Input: part model. Units: mm. Frame: model coordinates. A direction names the side the tool comes from. Coordinates: 2 decimals unless noted, no trailing zeros. Loops run counter-clockwise (first coordinate to the right, second up) from the corner with the lowest first, then second, coordinate; pieces in that order, holes last. Notation, with made-up numbers: (49, 57) - (92, 57) arc R22 cw to (92, 72) - close; hole circle Ø1 at (5.25, 78.5). An arc over 180 degrees is marked (long way). Use a Markdown table: item, result. Add a question column.
1. Ray query, L1, parallel to Z at x = 63, y = -8.25; L2, parallel to Y at x = 30.5, z = -8.5; L3, parallel to Z at x = -11.5, y = -5. Return the intervals inside material, ascending. Write a range as [from, to].
2. Section query C-C on z = 6. Return the cut outline in (x, y).
3. Contact query for flat-ended pins moving along their axis: P1, Ø3, axis at x = -13.5, y = -9.5, coming from the +Z side; P2, Ø1.5, axis at x = -59.09, z = -20.84, coming from the +Y side; P3, Ø7, axis at x = -11, y = -9, coming from the -Z side; P4, Ø17, axis at x = 19.5, z = -5, coming from the -Y side. Output: stop coordinate, or through.
4. Access query for faces 1 (the face through (10, -9, 16.801)), 2 (the face through (10, -6.35, 40)), 3 (the face through (10, 2, -22.216)). Directions: +Z, -Z, +X, -X, +Y, -Y. A direction counts if a zero-diameter tool reaches every point of the face in a straight line with its end or side. Return the directions, or none.
5. Section query B-B on y = -10.5. Return the cut outline in (x, z), then the cut area to 3 significant figures.
6. Section query A-A on x = 20.5. Return the cut outline in (y, z).
```python
from build123d import *

# Parameters (mm, degrees)
F0_W        = 142.24
F0_H        = 80.9625
F0_R        = 0.635
F1_DEPTH    = 6.35
F2_T1_DEPTH = 168.3682991577
F3_W        = 142.24
F3_H        = 9.525
F4_DEPTH    = 6.35


# Not quite as in the source:
# - a fillet or chamfer that OpenCascade refuses, or shapes differently, is made with other operations: its cross-section is extruded or revolved along the edge and cut away or added


with BuildPart() as f1:
    # F0 (on Front) → F1 (new body, symmetric)
    with BuildSketch(Plane.XZ):
        with Locations((10.6546021998, 18.2648575297)):
            Rectangle(F0_W, F0_H)
        with Locations((-59.0889267623, -20.8356846124)):
            Circle(F0_R, mode=Mode.SUBTRACT)
        with Locations((80.2197679877, -20.9288131446)):
            Circle(F0_R, mode=Mode.SUBTRACT)
        with Locations((-58.7598197162, 57.2748109698)):
            Circle(F0_R, mode=Mode.SUBTRACT)
        with Locations((80.3315266967, 57.7001310885)):
            Circle(F0_R, mode=Mode.SUBTRACT)
    extrude(amount=F1_DEPTH, both=True)

    # F2: chamfer of 5.08 on 2 edges, made by hand

    # F2_s2 → F2_t1 (cut)
    with BuildSketch(Plane.YZ.offset(-73.5295473791)):
        Polygon((-1.27, -22.2163924703), (-6.35, -17.1363924703), (-6.35, -22.2163924703), align=None)
        Polygon((-1.27, 58.7461075297), (-6.35, 53.6661075297), (-6.35, 58.7461075297), align=None)
    extrude(amount=F2_T1_DEPTH, mode=Mode.SUBTRACT)

    # F3 (on face) → F4 (join)
    with BuildSketch(Plane.XZ.offset(6.35)):
        with Locations((10.6546021998, 21.5639811352)):
            Rectangle(F3_W, F3_H)
    extrude(amount=F4_DEPTH)


solid = f1.part
```
Resolved:
| question | item | result |
|---|---|---|
| 1 | L1 | [16.8, 26.33] |
| 1 | L2 | [-6.35, 6.35] |
| 1 | L3 | [-18.49, 55.02] |
| 2 | outline | (-60.47, -6.35) - (81.77, -6.35) - (81.77, 6.35) - (-60.47, 6.35) - close |
| 3 | P1 | z = 26.33 |
| 3 | P2 | y = 6.35 |
| 3 | P3 | z = -17.99 |
| 3 | P4 | y = -6.35 |
| 4 | face 1 | -Z, +X, -X, -Y |
| 4 | face 2 | +Z, +X, -X, -Y |
| 4 | face 3 | -Z, +X, -X, +Y, -Y |
| 5 | outline | (-60.47, 16.8) - (81.77, 16.8) - (81.77, 26.33) - (-60.47, 26.33) - close |
| 5 | area | 1,350 mm² |
| 6 | outline | (-12.7, 16.8) - (-6.35, 16.8) - (-6.35, -17.14) - (-1.27, -22.22) - (6.35, -22.22) - (6.35, 58.75) - (-1.27, 58.75) - (-6.35, 53.67) - (-6.35, 26.33) - (-12.7, 26.33) - close |
